Autodesk Fusion 360 part; units mm, degrees
sketch "Sketch1" plane through (0, 0, 0) normal (0, 0, 1) x (1, 0, 0)
  line L0 (0, 0) -> (37, 0)
  line L1 (37, 0) -> (37, 30)
  line L2 (37, 30) -> (0, 30)
  line L3 (0, 30) -> (0, 0)
  circle A0 centre (12, 22.5) radius 2.75
  circle A1 centre (12, 7.5) radius 2.75
  line L4 (12, 30) -> (12, 0) construction
  line L5 (12, 15) -> (37, 15) construction
  circle A2 centre (12, 22.5) radius 6
  circle A3 centre (12, 7.5) radius 6
  line L6 (37, 21) -> (38.75, 21)
  line L7 (38.75, 21) -> (38.75, 9)
  line L8 (38.75, 9) -> (37, 9)
  line L9 (30, 21.1) -> (22, 21.1)
  arc A4 (22, 21.1) -> (22, 18.4) centre (22, 19.75) ccw
  line L10 (22, 18.4) -> (30, 18.4)
  arc A5 (30, 18.4) -> (30, 21.1) centre (30, 19.75) ccw
  line L11 (30, 19.75) -> (22, 19.75) construction
  line L12 (30, 19.75) -> (22, 19.75) construction
  line L13 (22, 11.6) -> (30, 11.6)
  arc A6 (30, 8.9) -> (30, 11.6) centre (30, 10.25) ccw
  arc A7 (22, 11.6) -> (22, 8.9) centre (22, 10.25) ccw
  line L14 (30, 8.9) -> (22, 8.9)
  line L15 (27.5, 25) -> (37, 25) construction
  line L16 (37, 25) -> (37, 5) construction
  line L17 (37, 5) -> (27.5, 5) construction
  line L18 (27.5, 5) -> (27.5, 25) construction
  line L19 (19.4, 22.35) -> (32.6, 22.35)
  line L20 (32.6, 22.35) -> (32.6, 17.15)
  line L21 (32.6, 17.15) -> (19.4, 17.15)
  line L22 (19.4, 17.15) -> (19.4, 22.35)
  line L23 (26, 19.75) -> (26, 22.35) construction
  line L24 (22, 19.75) -> (19.4, 19.75) construction
  line L25 (32.6, 12.85) -> (19.4, 12.85)
  line L26 (19.4, 12.85) -> (19.4, 7.65)
  line L27 (32.6, 7.65) -> (32.6, 12.85)
  line L28 (19.4, 7.65) -> (32.6, 7.65)
  line L29 (23.4, 22.35) -> (23.4, 30)
  line L30 (28.6, 30) -> (28.6, 22.35)
  line L31 (23.4, 7.65) -> (23.4, 0)
  line L32 (28.6, 0) -> (28.6, 7.65)
  dimension "d1" = 15
  dimension "d2" = 5.5
  dimension "d3" = 12
  dimension "d4" = 1.75
  dimension "d5" = 12
  dimension "d14" = 2.7
  dimension "d16" = 9.5
  dimension "d17" = 30
  dimension "d19" = 8
  dimension "d20" = 7
  dimension "d22" = 9.5
  dimension "d23" = 20
  dimension "d24" = 10
  dimension "d25" = 12
  dimension "d26" = 5.2
  dimension "d27" = 2.6
  dimension "d28" = 5.2
extrude "Extrude1" add sketch "Sketch1" along normal blind 11 contours L0 L1 L2 L3 L19 L20 L21 L22 L25 L26 L27 L28 L29 L30 L31 L32 | L0 L28 L31 L32 | L25 L26 L27 L28 | L2 L19 L29 L30 | L19 L20 L21 L22 | A2 | A3
extrude "Extrude2" add sketch "Sketch1" along normal blind 8 contours L1 L6 L7 L8
extrude "Extrude3" cut sketch "Sketch1" against normal blind 2 from surface at 11 contours A2 | A3
chamfer "Chamfer2" distance 1 angle 45 2 edges at (18.5, 0, 11) (18.5, 30, 11)
chamfer "Chamfer1" distance 4 angle 45 1 edges at (0, 15, 11)
ref_plane "WorkPlane1" through (18.5, 15, 5.5) normal (0, 0, 1) x (1, 0, 0)
extrude "Extrude4" cut sketch "Sketch1" along normal mid plane 1.8 from surface at 5.5 contours L0 L28 L31 L32 | L25 L26 L27 L28 | L2 L19 L29 L30 | L19 L20 L21 L22
extrude "Extrude5" add sketch "Sketch1" along normal blind 0.2 from surface at 6.4 contours L9 A4 L10 A5 | L13 A6 A7 L14
equation "d27 = d26 / 2"
equation "d28 = d26"
Design review of the part built by this model. Coordinates are the model's own, in mm. A direction names the side the tool comes from. Give positions to 0.01 mm unless a question says otherwise; leave off trailing zeros. Loops run counter-clockwise (first coordinate to the right, second up) from the corner with the lowest first, then second, coordinate; pieces in that order, holes last. Notation, with made-up numbers: M -18,36.25 L 24,36.25 A6 ccw 24,45.25 Z; hole C 89,89.5 d3. An arc over 180 degrees is marked long. Write item = value, one per line.
Q1. Insertion check: pin 1 (1.5 mm diameter, centred on x = 35, z = 8, fed in from -Y); pin 2 (7 mm diameter, centred on x = 12, y = 7.5, fed in from +Z); pin 3 (1.3 mm diameter, centred on x = 24, y = 10, fed in from +Z); pin 4 (0.5 mm diameter, centred on x = 26.5, z = 5.5, fed in from +Y). Each pin has a flat end and moves straight along its axis. Give the tip position at first contact, or say it passes through.
Output values:
pin_1 = 0
pin_2 = 9
pin_3 = 6.6
pin_4 = 17.15
Q2. We need section D-D (z = 1.25). Give the boundary of the cut face in (x, y), plus the area to 3 significant figures.
Output values:
outline = M 0,0 L 37,0 L 37,9 L 38.75,9 L 38.75,21 L 37,21 L 37,30 L 0,30 Z; hole C 12,7.5 d5.5; hole C 12,22.5 d5.5; hole M 22,8.9 L 30,8.9 A1.35 ccw 30,11.6 L 22,11.6 A1.35 ccw Z; hole M 22,18.4 L 30,18.4 A1.35 ccw 30,21.1 L 22,21.1 A1.35 ccw Z
area = 1,030 mm^2
Q3. Draft analysis for pull direction Z (two halves, no side actions). For faces 4 (the flat face through (24, 15, 11)), 5 (the flat face through (28.6, 4, 5)), 6 (the flat face through (38, 21, 4)), state which applies: +Z half, -Z half, draft (parallel to the pull), parting line (faces both ways), or undercut.
Output values:
face_4 = +Z half
face_5 = undercut
face_6 = draft
Q4. To check wall thickness, follow line 1 (Y direction, x = 12, z = 2.75); line 2 (Y direction, x = 26, z = 10); line 3 (X direction, y = 26.5, z = 5.25). State the ranges of each line that lie inside material, in increasing order. Write a range as [from, to].
Output values:
line_1 = [0, 4.75], [10.25, 19.75], [25.25, 30]
line_2 = [0, 8.9], [11.6, 18.4], [21.1, 30]
line_3 = [0, 23.4], [28.6, 37]
Q5. We need section B-B (z = 5.5). Give the boundary of the cut face in (x, y), plus the area to 3 significant figures.
Output values:
outline = M 0,0 L 23.4,0 L 23.4,7.65 L 19.4,7.65 L 19.4,12.85 L 32.6,12.85 L 32.6,7.65 L 28.6,7.65 L 28.6,0 L 37,0 L 37,9 L 38.75,9 L 38.75,21 L 37,21 L 37,30 L 28.6,30 L 28.6,22.35 L 32.6,22.35 L 32.6,17.15 L 19.4,17.15 L 19.4,22.35 L 23.4,22.35 L 23.4,30 L 0,30 Z; hole C 12,7.5 d5.5; hole C 12,22.5 d5.5
area = 867 mm^2
Q6. We need section A-A (x = 12). Give the boundary of the cut face in (y, z), plus the area to 3 significant figures.
Output values:
outline = M 0,0 L 4.75,0 L 4.75,9 L 1.5,9 L 1.5,11 L 1,11 L 0,10 Z; M 10.25,0 L 19.75,0 L 19.75,9 L 16.5,9 L 16.5,11 L 13.5,11 L 13.5,9 L 10.25,9 Z; M 25.25,0 L 30,0 L 30,10 L 29,11 L 28.5,11 L 28.5,9 L 25.25,9 Z
area = 182 mm^2
Q7. For faces 1 (the flat face through (26, 8.9, 2)), 2 (the cylindrical face through (31.35, 10.28, 8.77)), 3 (the flat face through (19.4, 10, 5)), list the 3-axis set-ups (+Z, -Z, +X, -X, +Y, -Y) from which the entire face can be reached by the end or side of a thin tool; tool diameter is ignored.
Output values:
face_1 = -Z
face_2 = +Z
face_3 = none
Q8. We need section C-C (y = 6.5). Give the boundary of the cut face in (x, z), plus the area to 3 significant figures.
Output values:
outline = M 0,0 L 9.44,0 L 9.44,9 L 6.08,9 L 6.08,11 L 4,11 L 0,7 Z; M 14.56,0 L 37,0 L 37,11 L 17.92,11 L 17.92,9 L 14.56,9 Z; hole M 23.4,4.6 L 28.6,4.6 L 28.6,6.4 L 23.4,6.4 Z
area = 320 mm^2
